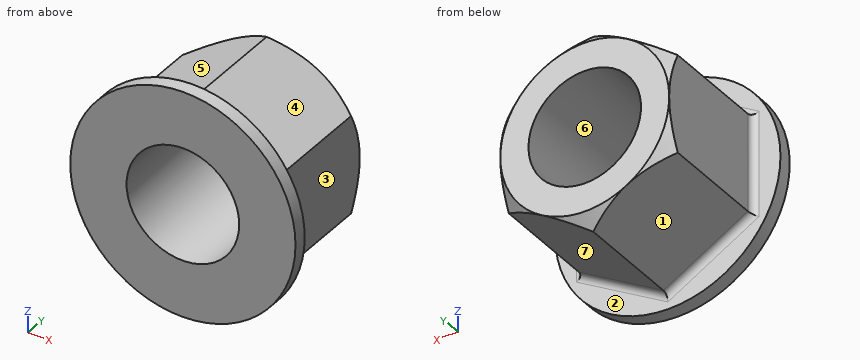
Autodesk Inventor part; units mm, degrees
ref_plane "YZ Plane" through (0, 0, 0) normal (1, 0, 0) x (0, 1, 0)
ref_plane "XZ Plane" through (0, 0, 0) normal (0, 1, 0) x (-1, 0, 0)
ref_plane "XY Plane" through (0, 0, 0) normal (0, 0, 1) x (1, 0, 0)
sketch "Sketch1" plane through (0, 0, 0) normal (0, 1, 0) x (-1, 0, 0)
  circle A0 centre (0, 0) radius 25.4
  dimension "d0" = 50.8
extrude "Extrusion1" add sketch "Sketch1" along normal blind 3.175
sketch "Sketch2" plane through (0, 3.175, 0) normal (0, 1, 0) x (1, 0, 0)
  circle A0 centre (0, 0) radius 19.05
  line L0 (-19.05, -10.9985) -> (-19.05, 10.9985)
  line L1 (-19.05, 10.9985) -> (0, 21.997)
  line L2 (0, 21.997) -> (19.05, 10.9985)
  line L3 (19.05, 10.9985) -> (19.05, -10.9985)
  line L4 (19.05, -10.9985) -> (0, -21.997)
  line L5 (0, -21.997) -> (-19.05, -10.9985)
  point P0 (-9.525, -16.4978)
  dimension "d3" = 38.1
extrude "Extrusion2" add sketch "Sketch2" along normal blind 28.575
sketch "Sketch3" plane through (0, 31.75, 0) normal (0, 1, 0) x (1, 0, 0)
  circle A0 centre (0, 0) radius 12.7
  dimension "d7" = 25.4
extrude "Extrusion3" cut sketch "Sketch3" against normal through all
thread "Thread1"
sketch "Sketch6" plane through (0, 31.75, 0) normal (0, 1, 0) x (1, 0, 0)
  circle A0 centre (0, 0) radius 19.05
  line L0 (-19.05, -10.9985) -> (0, -21.997)
extrude "Extrusion5" cut sketch "Sketch6" against normal through all draft 45 keep common part
fillet "Fillet2" radius 1.524 6 edges at (-19.05, 3.175, 0) (-9.525, 3.175, 16.4978) (9.525, 3.175, 16.4978) (-9.525, 3.175, -16.4978) (9.525, 3.175, -16.4978) (19.05, 3.175, 0)
properties part number "13_17"
Model file for the job. Use its own axes, mm. Face numbers are marked on the shaded views. A direction names the side the tool comes from. Round coordinates to 2 decimals unless told otherwise and drop trailing zeros. Write each loop counter-clockwise with the first axis right and the second up, starting at its lowest first coordinate (ties: lowest second). Pieces come first, ordered by that corner, then holes. Notation, with made-up numbers: M -3,15 L 43,15 A12 ccw 43,36 Z; hole C -3.5,40 d10. An arc over 180 degrees is marked long. Put each result on its own line as item: value.
Item 1: Cut at A-A (y = 22). List the corners of the cut face in (x, z), and give its area (3 significant figures).
Responses:
outline: M -19.05,-11 L 0,-22 L 19.05,-11 L 19.05,11 L 0,22 L -19.05,11 Z; hole C 0,0 d25.4
area: 750 mm²
Item 2: Flat gauge pins, fed straight in: P1, Ø3, axis at x = -18.5, z = 18.5, coming from the +Y side (3 decimals); P2, Ø11, axis at y = 18, z = -1, coming from the -X side; P3, Ø3, axis at x = -9, z = -3.5, coming from the +Y side; P4, Ø5, axis at y = 15.5, z = -4, coming from the +X side. Where does each tip first touch, or does it go through?
Responses:
P1: y = 3.175
P2: x = -19.05
P3: through
P4: x = 19.05
Item 3: Tool access for the marked faces 1, 2, 3 and 4: list every direction of +Z, -Z, +X, -X, +Y, -Y with a clear straight run to the whole face (end or side of a thin tool).
Responses:
face 1: -Z, -X, +Y
face 2: +Y
face 3: +Z, -Z, +X, +Y
face 4: +Z, +X, +Y
Item 4: Mould opens along Z. For the marked faces 5, 6 and 7 say: +Z half, -Z half, draft (parallel to the pull), parting line (faces both ways), or undercut.
Responses:
face 5: +Z half
face 6: undercut
face 7: -Z half
Item 5: Cut at B-B (y = 2). List the corners of the cut face in (x, z).
Responses:
outline: C 0,0 d50.8; hole C 0,0 d25.4
Item 6: Probe L1, parallel to X at y = 7, z = 0; L2, parallel to Z at x = 0, y = 7; L3, parallel to Z at x = 9, y = 29. List the from-to ranges inside material, lowest first. Write a range as from..to.
Responses:
L1: -19.05..-12.7, 12.7..19.05
L2: -22..-12.7, 12.7..22
L3: -16.8..-8.96, 8.96..16.8
